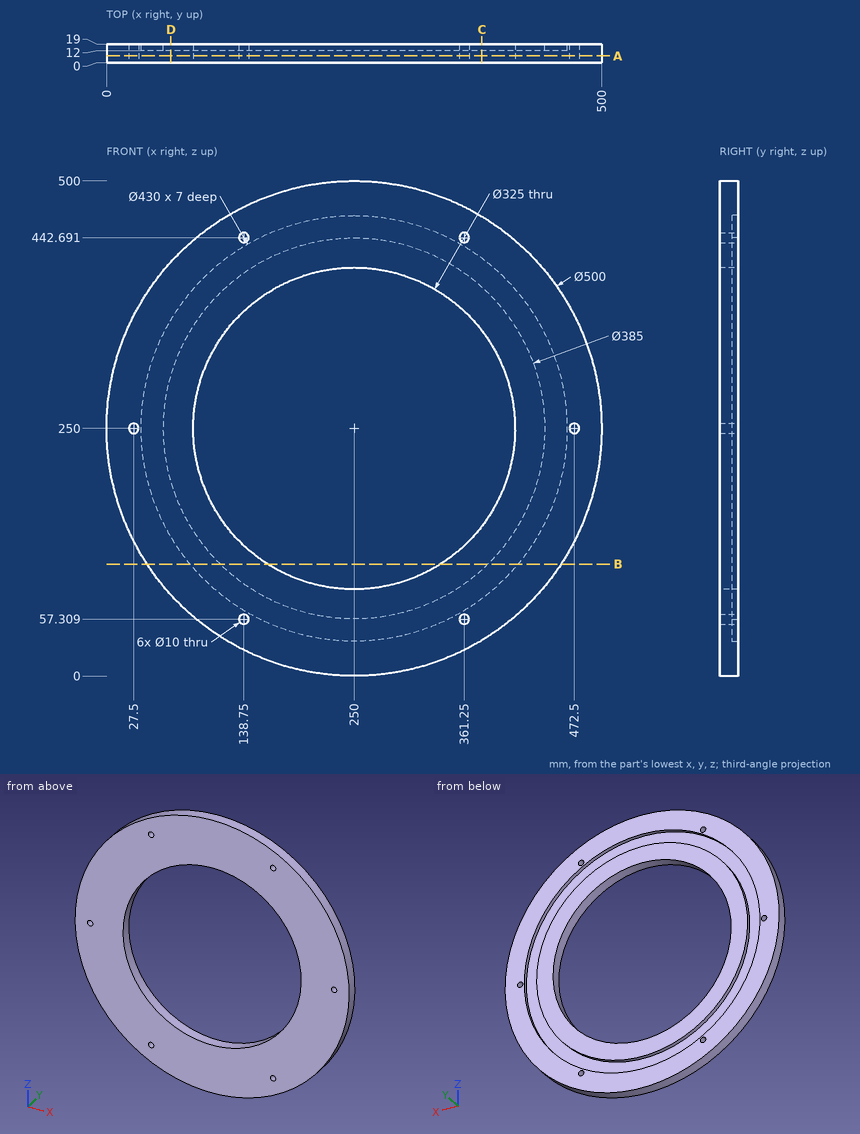
Can you work these out from the drawing? Everything is in mm from the part's minimum corner. Give positions to 0.01 mm unless a question says otherwise; leave off trailing zeros. Order: outer loops, then holes, each group sorted by start corner. A loop starts at its lowest first (then second) coordinate and runs counter-clockwise, first axis right, second up.
Item 1: If we section it at A-A, the plane y = 7: Write out the boundary of the cut face in (x, z).
Item 2: I'm going to push flat-ended pins straight in: pin 1 (11.5 mm diameter, centred on x = 138.75, z = 442.69, fed in from +Y); pin 2 (4 mm diameter, centred on y = 6, z = 235, fed in from -X); pin 3 (12 mm diameter, centred on x = 57.5, z = 172.5, fed in from +Y); pin 4 (3 mm diameter, centred on y = 5, z = 185, fed in from -X). Where does each tip first touch, or does it pass through?
Item 3: If we section it at C-C, the plane x = 379: Write out the boundary of the cut face in (y, z).
Item 4: If we section it at D-D, the plane x = 65: Write out the boundary of the cut face in (y, z) (1 decimal).
Item 5: If we section it at B-B, the plane z = 113: Write out the boundary of the cut face in (x, y).
Item 6: I need wall thicknesses on line 1 (X direction, y = 14.5, z = 250); line 2 (X direction, y = 14.75, z = 145.5) (1 decimal); line 3 (X direction, y = 10, z = 442). Which ranges of each line are inside material? Lowest first, please.
Values:
1. outline: circle Ø500 at (250, 250); hole circle Ø10 at (27.5, 250); hole circle Ø325 at (250, 250); hole circle Ø10 at (138.75, 57.31); hole circle Ø10 at (138.75, 442.69); hole circle Ø10 at (361.25, 57.31); hole circle Ø10 at (361.25, 442.69); hole circle Ø10 at (472.5, 250)
2. pin 1: stops at y = 19
2. pin 2: stops at x = 0.34
2. pin 3: stops at y = 12
2. pin 4: stops at x = 8.2
3. outline: (0, 35.85) - (19, 35.85) - (19, 78) - (12, 78) - (12, 107.12) - (19, 107.12) - (19, 151.18) - (0, 151.18) - close; (0, 348.82) - (19, 348.82) - (19, 392.88) - (12, 392.88) - (12, 422) - (19, 422) - (19, 464.15) - (0, 464.15) - close
4. outline: (0, 81.8) - (19, 81.8) - (19, 140.5) - (12, 140.5) - (12, 196.8) - (19, 196.8) - (19, 303.2) - (12, 303.2) - (12, 359.5) - (19, 359.5) - (19, 418.2) - (0, 418.2) - close
5. outline: (40.88, 0) - (162.61, 0) - (162.61, 19) - (114.77, 19) - (114.77, 12) - (84.3, 12) - (84.3, 19) - (40.88, 19) - close; (337.39, 0) - (459.12, 0) - (459.12, 19) - (415.7, 19) - (415.7, 12) - (385.23, 12) - (385.23, 19) - (337.39, 19) - close
6. line 1: x = 0 to 22.5, 32.5 to 35, 57.5 to 87.5, 412.5 to 442.5, 465 to 467.5, 477.5 to 500
6. line 2: x = 22.9 to 62.1, 88.3 to 125.6, 374.4 to 411.7, 437.9 to 477.1
6. line 3: x = 89.89 to 133.8, 143.7 to 356.3, 366.2 to 410.11
